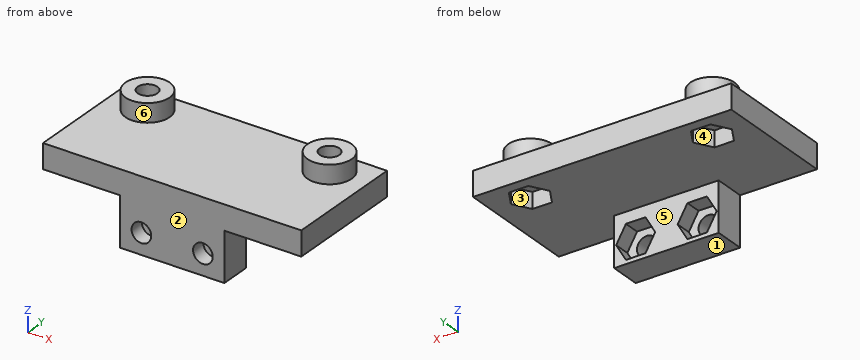
from build123d import *

# Parameters (mm, degrees)
SKETCH_1_W          = 42
SKETCH_1_H          = 20
SKETCH_1_R          = 3.6
EXTRUDE_1_DEPTH     = 4
SKETCH_1_3_R        = 3.6
SKETCH_1_3_R_2      = 1.6
EXTRUDE_2_DEPTH     = 7
CUT_EXTRUDE_3_DEPTH = 2.6
SKETCH_7_W          = 17
SKETCH_7_H          = 5
EXTRUDE_4_DEPTH     = 8
SKETCH_8_R          = 1.6
CUT_EXTRUDE_4_DEPTH = 6.6
CUT_EXTRUDE_5_DEPTH = 2.6


with BuildPart() as part:
    # Sketch 1 → Extrude 1 (new body)
    with BuildSketch(Plane.XY):
        with Locations((0, 5)):
            Rectangle(SKETCH_1_W, SKETCH_1_H)
        with Locations((-14.8, 10.5)):
            Circle(SKETCH_1_R, mode=Mode.SUBTRACT)
        with Locations((14.8, 10.5)):
            Circle(SKETCH_1_R, mode=Mode.SUBTRACT)
    extrude(amount=EXTRUDE_1_DEPTH)

    # Sketch 1_3 → Extrude 2 (add)
    # profile 1 of 2: a face of its own
    with BuildSketch(Plane.XY):
        with Locations((-14.8, 10.5)):
            Circle(SKETCH_1_3_R)
        with Locations((-14.8, 10.5)):
            Circle(SKETCH_1_3_R_2, mode=Mode.SUBTRACT)
    # profile 2 of 2: a face of its own
    with BuildSketch(Plane.XY):
        with Locations((14.8, 10.5)):
            Circle(SKETCH_1_3_R)
        with Locations((14.8, 10.5)):
            Circle(SKETCH_1_3_R_2, mode=Mode.SUBTRACT)
    extrude(amount=EXTRUDE_2_DEPTH)

    # Sketch 6 → Cut-Extrude 3 (cut)
    with BuildSketch(Plane(origin=(0, 0, 0), x_dir=(-1, 0, 0), z_dir=(0, 0, -1))):
        Polygon((-11.624573519, 10.5), (-13.21228676, 13.25), (-16.38771324, 13.25), (-17.975426481, 10.5), (-16.38771324, 7.75), (-13.21228676, 7.75), align=None)
        Polygon((17.975426481, 10.5), (16.38771324, 13.25), (13.21228676, 13.25), (11.624573519, 10.5), (13.21228676, 7.75), (16.38771324, 7.75), align=None)
    extrude(amount=-CUT_EXTRUDE_3_DEPTH, mode=Mode.SUBTRACT)

    # Sketch 7 → Extrude 4 (add)
    with BuildSketch(Plane(origin=(0, 0, 0), x_dir=(-1, 0, 0), z_dir=(0, 0, -1))):
        with Locations((0, -2.5)):
            Rectangle(SKETCH_7_W, SKETCH_7_H)
    extrude(amount=EXTRUDE_4_DEPTH)

    # Sketch 8 → Cut-Extrude 4 (cut)
    with BuildSketch(Plane(origin=(0, 0, 0), x_dir=(1, 0, 0), z_dir=(0, 1, 0))):
        with Locations(Location((-5, 4.6, 0), (0, 0, 180))):
            Circle(SKETCH_8_R)
        with Locations(Location((5, 4.6, 0), (0, 0, 180))):
            Circle(SKETCH_8_R)
    extrude(amount=-CUT_EXTRUDE_4_DEPTH, mode=Mode.SUBTRACT)

    # Sketch 9 → Cut-Extrude 5 (cut)
    with BuildSketch(Plane(origin=(0, 0, 0), x_dir=(1, 0, 0), z_dir=(0, 1, 0))):
        Polygon((1.824573519, 4.6), (3.41228676, 1.85), (6.58771324, 1.85), (8.175426481, 4.6), (6.58771324, 7.35), (3.41228676, 7.35), align=None)
        Polygon((-8.175426481, 4.6), (-6.58771324, 1.85), (-3.41228676, 1.85), (-1.824573519, 4.6), (-3.41228676, 7.35), (-6.58771324, 7.35), align=None)
    extrude(amount=-CUT_EXTRUDE_5_DEPTH, mode=Mode.SUBTRACT)


solid = part.part
Could you check a few things on this model? Use its own coordinates, in mm. Face numbers are marked on the shaded views. A direction names the side the tool comes from. Give positions to 0.01 mm unless a question says otherwise; leave off trailing zeros. Order: outer loops, then holes, each group sorted by start corner. A loop starts at its lowest first (then second) coordinate and runs counter-clockwise, first axis right, second up. Notation, with made-up numbers: (1.25, 71.5) - (8.25, 71.5) arc R29 cw to (8.25, 103.5) - close; hole circle Ø11 at (21.5, 58). An arc over 180 degrees is marked (long way). One line per question, with ' | ' between items. Start each with the question number.
Item 1: I'm going to push flat-ended pins straight in: pin 1 Ø1 at (x, y) = (14, 0.5) entering from +Z; pin 2 Ø1.5 at (y, z) = (-1.5, -3.5) entering from +X; pin 3 Ø1.6 at (x, z) = (-5.5, -3.5) entering from +Y. Where does each tip first touch, or does it pass through?
Item 2: Thinking about a two-plate mould opening in Y: for the marked faces 1, 2 and 3, which applies, pulls with the +Y half, pulls with the -Y half, needs draft (parallel to the pull), parting line crosses it, or undercut?
Item 3: I need wall thicknesses on probe 1 along Y at (x, z) = (14.8, 3.8); probe 2 along X at (y, z) = (10, 2.75); probe 3 along X at (y, z) = (-1.75, -0.5). Which ranges of each line are inside material? Lowest first, please. Write a range as [from, to].
Item 4: I want a section at C-C on z = 5. Write out the boundary of the cut face in (x, y).
Item 5: I want a section at B-B on y = -3. Write out the boundary of the cut face in (x, z), then the cut area to 3 significant figures.
Item 6: For the marked faces 4, 5 and 6, which set-ups out of +Z, -Z, +X, -X, +Y, -Y let a thin tool reach every point of the face, with its end or its side?
Item 7: I want a section at D-D on z = 3. Write out the boundary of the cut face in (x, y).
Item 8: I want a section at A-A on x = -14.8. Write out the boundary of the cut face in (y, z).
Verdict:
1) pin 1: z = 4 | pin 2: x = 8.5 | pin 3: y = -2.6
2) face 1: needs draft | face 2: pulls with the -Y half | face 3: undercut
3) probe 1: [-5, 8.9], [12.1, 15] | probe 2: [-21, -16.32], [-13.28, 13.28], [16.32, 21] | probe 3: [-8.5, 8.5]
4) outline: circle Ø7.2 at (-14.8, 10.5); circle Ø7.2 at (14.8, 10.5); hole circle Ø3.2 at (-14.8, 10.5); hole circle Ø3.2 at (14.8, 10.5)
5) outline: (-21, 0) - (-8.5, 0) - (-8.5, -8) - (8.5, -8) - (8.5, 0) - (21, 0) - (21, 4) - (-21, 4) - close; hole circle Ø3.2 at (-5, -4.6); hole circle Ø3.2 at (5, -4.6) | area: 288 mm^2
6) face 4: -Z | face 5: -Z, +X, -X, +Y | face 6: +Z
7) outline: (-21, -5) - (21, -5) - (21, 15) - (-21, 15) - close; hole circle Ø3.2 at (-14.8, 10.5); hole circle Ø3.2 at (14.8, 10.5)
8) outline: (-5, 0) - (7.75, 0) - (7.75, 2.6) - (8.9, 2.6) - (8.9, 7) - (6.9, 7) - (6.9, 4) - (-5, 4) - close; (12.1, 2.6) - (13.25, 2.6) - (13.25, 0) - (15, 0) - (15, 4) - (14.1, 4) - (14.1, 7) - (12.1, 7) - close
